Input: part model. Units: mm. Frame: model coordinates. Face numbers are marked on the shaded views. A direction names the side the tool comes from. Give positions to 0.01 mm unless a question says otherwise; leave off trailing zeros. Write each loop counter-clockwise with the first axis right and the second up, starting at its lowest first coordinate (ties: lowest second). Pieces come first, ordered by that corner, then holes. Notation, with made-up numbers: (65.25, 68.5) - (120.25, 68.5) arc R21 cw to (120.25, 86.5) - close; hole circle Ø11 at (-8, 22). An arc over 180 degrees is marked (long way). Answer as CSV lines item,"result".
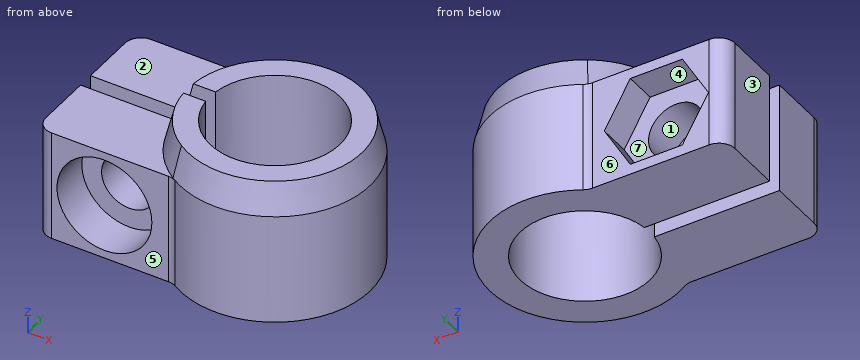
```python
from build123d import *

# Parameters (mm, degrees)
F1_DEPTH       = 9
F2_DEPTH       = 7
F7_D           = 3.5
F7_START       = 4.5
F7_CBORE_D     = 6
F7_CBORE_DEPTH = 2.5
F8_DEPTH       = 6.5
F9_SIZE2       = 1.99999
F9_SIZE        = 0.49999
F10_T1_DEPTH   = 7
F10_T3_DEPTH   = 7


# Not quite as in the source:
# - a fillet or chamfer that OpenCascade refuses, or shapes differently, is made with other operations: its cross-section is extruded or revolved along the edge and cut away or added
# - a fillet or chamfer is up to 0.001 mm smaller than in the source, because OpenCascade refuses the exact size


with BuildPart() as f1:
    # F0 (on Top) → F1 (new body)
    with BuildSketch(Plane.XY):
        with BuildLine():
            ThreePointArc((-4.0693979899, 0.5), (4.1, 0), (-4.0693979899, -0.5))
            Line((-4.0693979899, -0.5), (-5.9791303716, -0.5))
            ThreePointArc((-5.9791303716, -0.5), (-5.1638421749, -3.0552796914), (-3.3166247904, -5))
            ThreePointArc((-3.3166247904, -5), (6, 0), (-3.3166247904, 5))
            ThreePointArc((-3.3166247904, 5), (-5.1638421749, 3.0552796914), (-5.9791303716, 0.5))
            Line((-5.9791303716, 0.5), (-4.0693979899, 0.5))
        make_face()
    extrude(amount=F1_DEPTH)

    # F0 (on Top) → F2 (join)
    with BuildSketch(Plane.XY):
        with BuildLine():
            Line((-11.9791303716, 0.5), (-5.9791303716, 0.5))
            ThreePointArc((-5.9791303716, 0.5), (-5.1638421749, 3.0552796914), (-3.3166247904, 5))
            Line((-3.3166247904, 5), (-11.9791303716, 5))
            Line((-11.9791303716, 5), (-11.9791303716, 0.5))
        make_face()
        with BuildLine():
            ThreePointArc((-3.3166247904, -5), (-5.1638421749, -3.0552796914), (-5.9791303716, -0.5))
            Line((-5.9791303716, -0.5), (-11.9791303716, -0.5))
            Line((-11.9791303716, -0.5), (-11.9791303716, -5))
            Line((-11.9791303716, -5), (-3.3166247904, -5))
        make_face()
    extrude(amount=F2_DEPTH)

    # F7 (through all)
    # its depths count from where the whole tool has entered the part; down to there all is cleared
    with Locations(Plane.XZ.offset(9.5).offset(-F7_START)):
        with Locations((-7.647877581, 3.5)):
            CounterBoreHole(F7_D / 2, F7_CBORE_D / 2, F7_CBORE_DEPTH)

    # F6 (on offset) → F8 (cut)
    with BuildSketch(Plane(origin=(0, 9.5, 0), x_dir=(-1, 0, 0), z_dir=(0, 1, 0))):
        Polygon((6.0024293138, 0.65), (9.2933258481, 0.65), (10.9387741153, 3.5), (9.2933258481, 6.35), (6.0024293138, 6.35), (4.3569810466, 3.5), align=None)
    extrude(amount=-F8_DEPTH, mode=Mode.SUBTRACT)

    # F9 (size 0.5 and 2 in the source; OpenCascade refuses exactly that, so slightly less here)
    f9_edges = [f1.edges().sort_by_distance(p)[0] for p in [
        (5.400488, -2.614332, 9),
    ]]
    f9_side = f1.faces().sort_by_distance((-5.017914, 2.968938, 9))[0]
    chamfer(f9_edges, length=F9_SIZE, length2=F9_SIZE2, reference=f9_side)

    # F10: fillet of radius 1 on 4 edges, made by hand

    # F10_s2 → F10_t1 (join)
    with BuildSketch(Plane.XY):
        with BuildLine():
            ThreePointArc((-3.0904725218, -5.1428571429), (-3.3382900336, -5.0363758883), (-3.6055512755, -5))
            Line((-3.6055512755, -5), (-3.6055512755, -4.98))
            Line((-3.6055512755, -4.98), (-3.3166247904, -4.98))
            Line((-3.3166247904, -4.98), (-3.3055693744, -4.9833333333))
            ThreePointArc((-3.3055693744, -4.9833333333), (-3.1936637184, -5.0557800638), (-3.0801709468, -5.1257142857))
            Line((-3.0801709468, -5.1257142857), (-3.0904725218, -5.1428571429))
        make_face()
        with BuildLine():
            ThreePointArc((-3.0904725218, 5.1428571429), (-3.3382900336, 5.0363758883), (-3.6055512755, 5))
            Line((-3.6055512755, 5), (-3.6055512755, 4.98))
            Line((-3.6055512755, 4.98), (-3.3166247904, 4.98))
            Line((-3.3166247904, 4.98), (-3.3055693744, 4.9833333333))
            ThreePointArc((-3.3055693744, 4.9833333333), (-3.1936637184, 5.0557800638), (-3.0801709468, 5.1257142857))
            Line((-3.0801709468, 5.1257142857), (-3.0904725218, 5.1428571429))
        make_face()
    extrude(amount=F10_T1_DEPTH)

    # F10_s4 → F10_t3 (cut)
    with BuildSketch(Plane.XY):
        with BuildLine():
            ThreePointArc((-10.9791303716, -5), (-11.6862371527, -4.7071067812), (-11.9791303716, -4))
            Line((-11.9791303716, -4), (-11.9991303716, -4))
            Line((-11.9991303716, -4), (-11.9991303716, -5.02))
            Line((-11.9991303716, -5.02), (-10.9791303716, -5.02))
            Line((-10.9791303716, -5.02), (-10.9791303716, -5))
        make_face()
        with BuildLine():
            ThreePointArc((-11.9791303716, 4), (-11.6862371527, 4.7071067812), (-10.9791303716, 5))
            Line((-10.9791303716, 5), (-10.9791303716, 5.02))
            Line((-10.9791303716, 5.02), (-11.9991303716, 5.02))
            Line((-11.9991303716, 5.02), (-11.9991303716, 4))
            Line((-11.9991303716, 4), (-11.9791303716, 4))
        make_face()
    extrude(amount=F10_T3_DEPTH, mode=Mode.SUBTRACT)


solid = f1.part
```
Item 1: Cut plane C-C on y = 0. Return the cut outline in (x, z).
The answers:
outline,"(4.1, 0) - (6, 0) - (6, 7) - (5.5, 9) - (4.1, 9) - close"
Item 2: Ray query, line 1 (Y direction, x = -11, z = 0.5); line 2 (X direction, y = -1.25, z = 5); line 3 (Y direction, x = 0, z = 4.5). Return the intervals inside material, ascending. Write a range as from..to.
The answers:
line 1,"-5..-0.5, 0.5..5"
line 2,"-11.98..-8.55, -6.75..-3.9, 3.9..5.87"
line 3,"-6..-4.1, 4.1..6"
Item 3: Contact query for flat-ended pins moving along their axis: pin 1 (1 mm diameter, centred on x = -5, y = 4.5, fed in from -Z); pin 2 (1.6 mm diameter, centred on x = -8.5, y = 4, fed in from +Z); pin 3 (1.5 mm diameter, centred on y = 3.5, z = 8, fed in from -X); pin 4 (4 mm diameter, centred on x = -7.65, z = 3.5, fed in from +Y). Output: stop coordinate, or through.
The answers:
pin 1,"z = 0"
pin 2,"z = 7"
pin 3,"x = -5.1"
pin 4,"y = 3"
Item 4: Cut plane A-A on x = 0. Return the cut outline in (y, z), plus the area to 3 significant figures.
The answers:
outline,"(-6, 0) - (-4.1, 0) - (-4.1, 9) - (-5.5, 9) - (-6, 7) - close; (4.1, 0) - (6, 0) - (6, 7) - (5.5, 9) - (4.1, 9) - close"
area,"33.2 mm²"
Item 5: Mould query, pull axis Z, two halves, no side actions, for the marked faces 1, 2, 3 and 4. Classes: +Z half, -Z half, draft (parallel to the pull), parting line (faces both ways), or undercut.
The answers:
face 1,"undercut"
face 2,"+Z half"
face 3,"draft"
face 4,"undercut"
Item 6: Reachability of the marked faces 5, 6 and 7 from +Z, -Z, +X, -X, +Y, -Y: full face, straight path, thin tool, end or side. Return the list, or none.
The answers:
face 5,"+Z, -Z, -X, -Y"
face 6,"+Z, -Z, -X, +Y"
face 7,"+Y"
Item 7: Cut plane D-D on y = -1.75. Count the separate pieces of the cut face and the enclosed holes in it, plus the area to 3 significant figures.
The answers:
separate pieces,"2"
enclosed holes,"1"
area,"69.6 mm²"
Item 8: Cut plane B-B on z = 5. Return the cut outline in (x, y).
The answers:
outline,"(-11.98, -4) arc R1 ccw to (-10.98, -5) - (-10.25, -5) - (-10.25, -2.5) - (-8.55, -2.5) - (-8.55, -0.5) - (-11.98, -0.5) - close; (-11.98, 0.5) - (-8.55, 0.5) - (-8.55, 3) - (-10.07, 3) - (-10.07, 5) - (-10.98, 5) arc R1 ccw to (-11.98, 4) - close; (-6.75, -2.5) - (-5.05, -2.5) - (-5.05, -5) - (-3.61, -5) arc R1 cw to (-3.09, -5.14) arc R6 ccw (long way) to (-3.09, 5.14) arc R1 cw to (-3.61, 5) - (-5.22, 5) - (-5.22, 3) - (-6.75, 3) - (-6.75, 0.5) - (-4.07, 0.5) arc R4.1 cw (long way) to (-4.07, -0.5) - (-6.75, -0.5) - close"
